```python
from build123d import *

# Parameters (mm, degrees)
POCKET_DEPTH = 1.25


with BuildPart() as part:
    # Sketch (on DatumPlane) → Revolution (revolve)
    with BuildSketch(Plane.YZ):
        Polygon((0, 0), (0, -2.5), (19.75, -2.5), (20, -2.25), (20, -0.25), (19.75, 0), align=None)
    revolve(axis=Axis((0, 0, 0), (0, 0, 1)))

    # Sketch005 → Pocket (cut)
    with BuildSketch(Plane.XY):
        with BuildLine():
            add(Edge.make_bspline(
                [(-9.952404, 3.739768), (-8.508605, 0.536828), (-8.949612, -2.784858), (-10.937289, -3.681478)],
                knots=[0, 0, 0, 0, 1, 1, 1, 1], degree=3))
            add(Edge.make_bspline(
                [(-10.937289, -3.681478), (-12.92503, -4.578098), (-15.706774, -2.709293), (-17.150447, 0.493013)],
                knots=[0, 0, 0, 0, 1, 1, 1, 1], degree=3))
            add(Edge.make_bspline(
                [(-17.150447, 0.493013), (-18.594246, 3.695318), (-18.153302, 7.01732), (-16.165562, 7.913813)],
                knots=[0, 0, 0, 0, 1, 1, 1, 1], degree=3))
            add(Edge.make_bspline(
                [(-16.165562, 7.913813), (-14.177821, 8.810052), (-11.396204, 6.941184), (-9.952404, 3.739768)],
                knots=[0, 0, 0, 0, 1, 1, 1, 1], degree=3))
        make_face()
        with BuildLine():
            add(Edge.make_bspline(
                [(9.695893, 3.739768), (8.25203, 0.536828), (8.693037, -2.784858), (10.680905, -3.681478)],
                knots=[0, 0, 0, 0, 1, 1, 1, 1], degree=3))
            add(Edge.make_bspline(
                [(10.680905, -3.681478), (12.668645, -4.578098), (15.450136, -2.709293), (16.894126, 0.493013)],
                knots=[0, 0, 0, 0, 1, 1, 1, 1], degree=3))
            add(Edge.make_bspline(
                [(16.894126, 0.493013), (18.337735, 3.695318), (17.896727, 7.01732), (15.90905, 7.913813)],
                knots=[0, 0, 0, 0, 1, 1, 1, 1], degree=3))
            add(Edge.make_bspline(
                [(15.90905, 7.913813), (13.921437, 8.810052), (11.139692, 6.941184), (9.695893, 3.739768)],
                knots=[0, 0, 0, 0, 1, 1, 1, 1], degree=3))
        make_face()
        with BuildLine():
            add(Edge.make_bspline(
                [(-1.503564, 10.159173), (-0.763484, 6.725792), (-1.8916, 3.570223), (-4.023162, 3.110483)],
                knots=[0, 0, 0, 0, 1, 1, 1, 1], degree=3))
            add(Edge.make_bspline(
                [(-4.023162, 3.110483), (-6.154565, 2.651378), (-8.482443, 5.062473), (-9.222408, 8.495537)],
                knots=[0, 0, 0, 0, 1, 1, 1, 1], degree=3))
            add(Edge.make_bspline(
                [(-9.222408, 8.495537), (-9.962374, 11.928855), (-8.834296, 15.084551), (-6.702779, 15.543846)],
                knots=[0, 0, 0, 0, 1, 1, 1, 1], degree=3))
            add(Edge.make_bspline(
                [(-6.702779, 15.543846), (-4.571281, 16.003332), (-2.243517, 13.592555), (-1.503564, 10.159173)],
                knots=[0, 0, 0, 0, 1, 1, 1, 1], degree=3))
        make_face()
        with BuildLine():
            add(Edge.make_bspline(
                [(1.194043, 10.156252), (0.454611, 6.722934), (1.581926, 3.567048), (3.713329, 3.107943)],
                knots=[0, 0, 0, 0, 1, 1, 1, 1], degree=3))
            add(Edge.make_bspline(
                [(3.713329, 3.107943), (5.844872, 2.648203), (8.172655, 5.059298), (8.912557, 8.492552)],
                knots=[0, 0, 0, 0, 1, 1, 1, 1], degree=3))
            add(Edge.make_bspline(
                [(8.912557, 8.492552), (9.652586, 11.925934), (8.524635, 15.08163), (6.393004, 15.540925)],
                knots=[0, 0, 0, 0, 1, 1, 1, 1], degree=3))
            add(Edge.make_bspline(
                [(6.393004, 15.540925), (4.261448, 16.000284), (1.933716, 13.589634), (1.194043, 10.156252)],
                knots=[0, 0, 0, 0, 1, 1, 1, 1], degree=3))
        make_face()
        with BuildLine():
            add(Edge.make_bspline(
                [(-4.171396, -1.318008), (-4.691613, -2.216533), (-7.102321, -5.190873), (-8.769717, -6.205603)],
                knots=[0, 0, 0, 0, 1, 1, 1, 1], degree=3))
            add(Edge.make_bspline(
                [(-8.769717, -6.205603), (-10.436973, -7.220333), (-12.503009, -8.706233), (-12.156299, -12.118088)],
                knots=[0, 0, 0, 0, 1, 1, 1, 1], degree=3))
            add(Edge.make_bspline(
                [(-12.156299, -12.118088), (-11.809779, -15.530578), (-8.309786, -16.991078), (-6.005708, -16.861538)],
                knots=[0, 0, 0, 0, 1, 1, 1, 1], degree=3))
            add(Edge.make_bspline(
                [(-6.005708, -16.861538), (-3.701502, -16.732633), (0.642698, -16.308453), (3.744273, -16.738348)],
                knots=[0, 0, 0, 0, 1, 1, 1, 1], degree=3))
            add(Edge.make_bspline(
                [(3.744273, -16.738348), (6.845695, -17.168243), (10.760153, -16.842488), (11.676839, -13.575413)],
                knots=[0, 0, 0, 0, 1, 1, 1, 1], degree=3))
            add(Edge.make_bspline(
                [(11.676839, -13.575413), (12.593525, -10.308338), (10.543364, -8.226808), (8.943545, -7.045708)],
                knots=[0, 0, 0, 0, 1, 1, 1, 1], degree=3))
            add(Edge.make_bspline(
                [(8.943545, -7.045708), (7.343789, -5.865243), (4.672217, -2.334008), (3.849137, -0.712853)],
                knots=[0, 0, 0, 0, 1, 1, 1, 1], degree=3))
            add(Edge.make_bspline(
                [(3.849137, -0.712853), (3.026177, 0.907668), (-1.162715, 3.875658), (-4.171396, -1.318008)],
                knots=[0, 0, 0, 0, 1, 1, 1, 1], degree=3))
        make_face()
    extrude(amount=-POCKET_DEPTH, mode=Mode.SUBTRACT)


solid = part.part
```
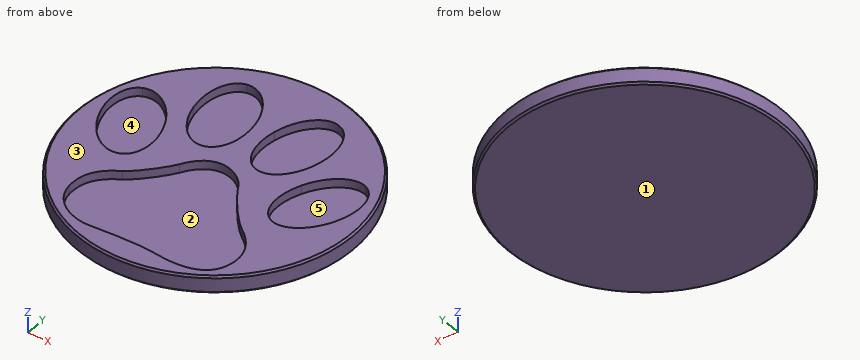
For this review, take the finished solid that the model builds, in its own axes (mm). Face numbers are marked on the shaded views. A direction names the side the tool comes from. Round coordinates to 2 decimals unless told otherwise and drop trailing zeros.
(1) Clearance check with flat-ended pins moving along their axes: P1, Ø4, axis at x = -5.5, y = 8.5, coming from the +Z side; P2, Ø1.5, axis at x = -7.5, z = -2, coming from the +Y side. State where each tip first meets the part, or that it passes through.
Returned:
P1: stops at z = -1.25
P2: stops at y = 18.83
(2) Mouldability with a two-part tool opening along X and no side actions: class the marked faces 3, 4 and 5 as released by +X, released by -X, zero draft, split by the parting line, or undercut.
Returned:
face 3: zero draft
face 4: undercut
face 5: undercut
(3) Tool access review of the marked faces 1 and 2: name each direction out of +Z, -Z, +X, -X, +Y, -Y from which nothing blocks a thin tool from reaching the whole face with its end or side.
Returned:
face 1: -Z, +X, -X, +Y, -Y
face 2: +Z
(4) Wall thickness on line 1 along Y through (x, z) = (9.5, -0.6); line 2 along Y through (x, z) = (-8, -0.3); line 3 along X through (y, z) = (3.5, -0.7): over which ranges is each line inside the solid? List them lowest first.
Returned:
line 1: y = -17.6 to -16.17, -7.48 to -2.62, 3.28 to 17.6
line 2: y = -18.33 to -16.63, -5.65 to 5.44, 14.83 to 18.33
line 3: x = -19.69 to -17.97, -9.85 to -6.09, -3.12 to 2.81, 5.78 to 9.59, 17.71 to 19.69
(5) We need section A-A (z = -0.7). State how many separate pieces and enclosed holes the cut face has, plus the area to 3 significant figures.
Returned:
separate pieces: 1
enclosed holes: 5
area: 634 mm2
